```python
from build123d import *

# Parameters (mm, degrees)
F0_R     = 2.5
F1_DEPTH = 5


# Not quite as in the source:
# - a feature names something its author has since deleted; it is built from what else it names


with BuildPart() as f1:
    # F0 (on Front) → F1 (new body)
    with BuildSketch(Plane.XZ):
        with BuildLine():
            ThreePointArc((19.4855715851, -11.25), (21.7333310915, -5.8234285148), (22.5, 0))
            ThreePointArc((22.5, 0), (22.4630219271, 1.2894362728), (22.3522092532, 2.5746342462))
            ThreePointArc((22.3522092532, 2.5746342462), (22.2651615708, 3.2423109389), (22.1581744428, 3.9070839975))
            ThreePointArc((22.1581744428, 3.9070839975), (19.8134723767, 10.6619094152), (15.4678426969, 16.3400074145))
            ThreePointArc((15.4678426969, 16.3400074145), (14.9719859982, 16.795524263), (14.4627212179, 17.2359999702))
            ThreePointArc((14.4627212179, 17.2359999702), (8.3246571453, 20.9033510092), (1.3459006368, 22.4597095145))
            ThreePointArc((1.3459006368, 22.4597095145), (0.6732517819, 22.489925123), (0, 22.5))
            ThreePointArc((0, 22.5), (-7.0593576826, 21.363882351), (-13.4058032893, 18.0702639208))
            ThreePointArc((-13.4058032893, 18.0702639208), (-13.9405044255, 17.6610400702), (-14.4627212179, 17.2359999702))
            ThreePointArc((-14.4627212179, 17.2359999702), (-19.1402205948, 11.8280157078), (-21.8847828674, 5.22554101))
            ThreePointArc((-21.8847828674, 5.22554101), (-22.0313436808, 4.568358088), (-22.1581744428, 3.9070839975))
            ThreePointArc((-22.1581744428, 3.9070839975), (-22.2651615708, -3.2423109389), (-20.1236293196, -10.0642706148))
            ThreePointArc((-20.1236293196, -10.0642706148), (-19.8134723767, -10.6619094152), (-19.4855715851, -11.25))
            ThreePointArc((-19.4855715851, -11.25), (-14.9719859982, -16.795524263), (-8.9464059639, -20.6448981671))
            ThreePointArc((-8.9464059639, -20.6448981671), (-8.3246571453, -20.9033510092), (-7.6954532248, -21.1430839677))
            ThreePointArc((-7.6954532248, -21.1430839677), (-0.6732517819, -22.489925123), (6.4169401705, -21.5655484245))
            ThreePointArc((6.4169401705, -21.5655484245), (7.0593576826, -21.363882351), (7.6954532248, -21.1430839677))
            ThreePointArc((7.6954532248, -21.1430839677), (13.9405044255, -17.6610400702), (18.7777286828, -12.3954388997))
            ThreePointArc((18.7777286828, -12.3954388997), (19.1402205948, -11.8280157078), (19.4855715851, -11.25))
        make_face()
        Circle(F0_R, mode=Mode.SUBTRACT)
        with BuildLine():
            ThreePointArc((-13.4058032893, 18.0702639208), (-7.0593576826, 21.363882351), (0, 22.5))
            ThreePointArc((0, 22.5), (1.2893242582, 25.1998179584), (3.7992770591, 26.8281640483))
            Line((3.7992770591, 26.8281640483), (-5.477073051, 23.9523583039))
            Line((-5.477073051, 23.9523583039), (-13.4058032893, 18.0702639208))
        make_face()
        with BuildLine():
            ThreePointArc((-21.8847828674, 5.22554101), (-19.1402205948, 11.8280157078), (-14.4627212179, 17.2359999702))
            ThreePointArc((-14.4627212179, 17.2359999702), (-15.2104510666, 20.1329421727), (-14.3343963619, 22.9936942077))
            Line((-14.3343963619, 22.9936942077), (-19.5919605158, 14.8279762838))
            Line((-19.5919605158, 14.8279762838), (-21.8847828674, 5.22554101))
        make_face()
        with BuildLine():
            Line((-24.5395519148, -1.2345806341), (-20.1236293196, -10.0642706148))
            ThreePointArc((-20.1236293196, -10.0642706148), (-22.2651615708, -3.2423109389), (-22.1581744428, 3.9070839975))
            ThreePointArc((-22.1581744428, 3.9070839975), (-24.5930872921, 5.6456389916), (-25.7608464161, 8.4002193008))
            Line((-25.7608464161, 8.4002193008), (-24.5395519148, -1.2345806341))
        make_face()
        with BuildLine():
            Line((-18.0048142462, -16.7194635525), (-8.9464059639, -20.6448981671))
            ThreePointArc((-8.9464059639, -20.6448981671), (-14.9719859982, -16.795524263), (-19.4855715851, -11.25))
            ThreePointArc((-19.4855715851, -11.25), (-22.4683446518, -11.4833214179), (-25.1335101323, -10.1238115749))
            Line((-25.1335101323, -10.1238115749), (-18.0048142462, -16.7194635525))
        make_face()
        with BuildLine():
            Line((-3.0454238906, -24.3811236585), (6.4169401705, -21.5655484245))
            ThreePointArc((6.4169401705, -21.5655484245), (-0.6732517819, -22.489925123), (-7.6954532248, -21.1430839677))
            ThreePointArc((-7.6954532248, -21.1430839677), (-9.8304138412, -23.2391081131), (-12.7459251298, -23.9107985011))
            Line((-12.7459251298, -23.9107985011), (-3.0454238906, -24.3811236585))
        make_face()
        with BuildLine():
            ThreePointArc((22.3522092532, 2.5746342462), (22.4630219271, 1.2894362728), (22.5, 0))
            ThreePointArc((22.5, 0), (21.7333310915, -5.8234285148), (19.4855715851, -11.25))
            ThreePointArc((19.4855715851, -11.25), (21.1790203936, -13.7164965405), (21.3342330732, -16.7043524734))
            Line((21.3342330732, -16.7043524734), (23.4818872972, -7.2328947514))
            Line((23.4818872972, -7.2328947514), (22.3522092532, 2.5746342462))
        make_face()
        with BuildLine():
            Line((13.3389541496, -20.6345850387), (18.7777286828, -12.3954388997))
            ThreePointArc((18.7777286828, -12.3954388997), (13.9405044255, -17.6610400702), (7.6954532248, -21.1430839677))
            ThreePointArc((7.6954532248, -21.1430839677), (7.4072768587, -24.1210578483), (5.6056198962, -26.5096570697))
            Line((5.6056198962, -26.5096570697), (13.3389541496, -20.6345850387))
        make_face()
        with BuildLine():
            ThreePointArc((1.3459006368, 22.4597095145), (8.3246571453, 20.9033510092), (14.4627212179, 17.2359999702))
            ThreePointArc((14.4627212179, 17.2359999702), (17.1858104334, 18.4754188566), (20.1552265199, 18.1094377689))
            Line((20.1552265199, 18.1094377689), (11.2005977653, 21.8691656728))
            Line((11.2005977653, 21.8691656728), (1.3459006368, 22.4597095145))
        make_face()
        with BuildLine():
            ThreePointArc((15.4678426969, 16.3400074145), (19.8134723767, 10.6619094152), (22.1581744428, 3.9070839975))
            ThreePointArc((22.1581744428, 3.9070839975), (25.0408649078, 3.1061659404), (27.0803214916, 0.9171042935))
            Line((27.0803214916, 0.9171042935), (22.6373844064, 9.5531473747))
            Line((22.6373844064, 9.5531473747), (15.4678426969, 16.3400074145))
        make_face()
    extrude(amount=F1_DEPTH)


solid = f1.part
```
The listing builds one solid part. Answer for the finished solid, in the listing's coordinates (mm). A direction names the side the tool comes from. Coordinates: 2 decimals unless noted, no trailing zeros. Loops run counter-clockwise (first coordinate to the right, second up) from the corner with the lowest first, then second, coordinate; pieces in that order, holes last. Notation, with made-up numbers: M 4,63.5 L 48,63.5 A27 cw 48,99.5 Z; hole C -18,60 d8. An arc over 180 degrees is marked long. Answer as CSV lines item,"result". Start each with the question number.
(1) The part is cut by section D-D (z = 13). Give the vertices of the cut face in (x, y).
(2) The part is cut by section B-B (z = 0). Give the vertices of the cut face in (x, y), and give its area (3 significant figures).
(3) The mould has two halves that part along Z. Classify faces 1 (the cylindrical face through (7.423, -2.465, -24.081)), 2 (the cylindrical face through (17.14, -2.46, 18.47)), 3 (the flat face through (22.4, -2.5, -12)), 4 (the flat face through (24.89, -2.465, 5.175)): pulls with the +Z half, pulls with the -Z half, needs draft (parallel to the pull), parting line crosses it, or undercut.
(4) For faces 5 (the flat face through (16, -2.5, -16.6)), 6 (the flat face through (-22.36, -2.46, -5.59)), 7 (the flat face through (6.34, -2.46, 22.16)), 8 (the flat face through (-9.39, -2.46, 21.05)), determine the directions among +Z, -Z, +X, -X, +Y, -Y from which every point of the face is accessible in a straight line to the end or side of a thin tool.
(5) Given pin 1 (3 mm diameter, centred on x = -20, y = -4.5, fed in from +Z); pin 2 (1.5 mm diameter, centred on y = -3.5, z = -5.5, fed in from -X), each flat-ended and moving along its own axis, determine where each tip first touches the part or whether it passes through.
(6) The part is cut by section C-C (x = 4.5). Give the vertices of the cut face in (y, z).
(7) The part is cut by section A-A (z = 20.5). Give the vertices of the cut face in (x, y).
(8) Find the intervals of material crossed by L1, parallel to X at y = -0.2, z = 6; L2, parallel to Z at x = -0.5, y = -2.1; L3, parallel to X at y = -4.05, z = -14, in increasing order. Write a range as [from, to].
Determined:
1,outline,"M -20.03,-5 L 19,-5 L 19,0 L -20.03,0 Z"
2,outline,"M -24.7,-5 L -2.5,-5 L -2.5,0 L -24.7,0 Z; M 2.5,-5 L 22.65,-5 L 22.65,0 L 2.5,0 Z"
2,area,"212 mm2"
3,face 1,"undercut"
3,face 2,"undercut"
3,face 3,"pulls with the -Z half"
3,face 4,"pulls with the +Z half"
4,face 5,"-Z, +Y, -Y"
4,face 6,"-X, +Y, -Y"
4,face 7,"+X, +Y, -Y"
4,face 8,"+Z, +Y, -Y"
5,pin 1,"z = 16.52"
5,pin 2,"x = -22.78"
6,outline,"M -5,-22.14 L 0,-22.14 L 0,22.27 L -5,22.27 Z"
7,outline,"M -15.94,-5 L -15.19,-5 L -15.19,0 L -15.94,0 Z; M -10.13,-5 L 14.46,-5 L 14.46,0 L -10.13,0 Z"
8,L1,"[-25.46, -24.85], [-21.7, 24.47]"
8,L2,"[-23.62, -2.45], [2.45, 25.5]"
8,L3,"[-20.94, 17.72], [21.27, 21.95]"
